from build123d import *

# Parameters (mm, degrees)
SKETCH1_W               = 107.35
SKETCH1_H               = 69.35
BOSS_EXTRUDE1_DEPTH     = 1.5875
CUT_EXTRUDE2_DEPTH      = 64.920899605
CUT_EXTRUDE2_DEPTH_BACK = 64.920899605
SKETCH2_R               = 1.5
SKETCH2_W               = 101
SKETCH2_H               = 42
SKETCH3_W               = 107.35
SKETCH3_H               = 69.35
SKETCH3_W_2             = 101
SKETCH3_H_2             = 63
BOSS_EXTRUDE2_DEPTH     = 40
SKETCH5_R               = 3.571875
CUT_EXTRUDE3_DEPTH      = 25.4
CUT_EXTRUDE4_DEPTH      = 121.232683914
SKETCH10_W              = 47.370876146
SKETCH10_H              = 31.5
CUT_EXTRUDE5_DEPTH      = 25.4
FILLET1_R               = 1.5


with BuildPart() as part:
    # Sketch1 → Boss-Extrude1 (new, symmetric)
    with BuildSketch(Plane.XY):
        Rectangle(SKETCH1_W, SKETCH1_H)
    extrude(amount=BOSS_EXTRUDE1_DEPTH, both=True)

    # Sketch2 → Cut-Extrude2 (cut, two sides: drawn at the far end of the back side and taken through both)
    with BuildSketch(Plane.XY.offset(-CUT_EXTRUDE2_DEPTH_BACK)):
        with Locations((-46.5, 27.5)):
            Circle(SKETCH2_R)
        with Locations((46.5, 27.5)):
            Circle(SKETCH2_R)
        with Locations((46.5, -27.5)):
            Circle(SKETCH2_R)
        with Locations((-46.5, -27.5)):
            Circle(SKETCH2_R)
        Rectangle(SKETCH2_W, SKETCH2_H)
    extrude(amount=CUT_EXTRUDE2_DEPTH + CUT_EXTRUDE2_DEPTH_BACK, mode=Mode.SUBTRACT)

    # Sketch3 → Boss-Extrude2 (add)
    with BuildSketch(Plane(origin=(0, 0, -1.5875), x_dir=(-1, 0, 0), z_dir=(0, 0, -1))):
        Rectangle(SKETCH3_W, SKETCH3_H)
        Rectangle(SKETCH3_W_2, SKETCH3_H_2, mode=Mode.SUBTRACT)
    extrude(amount=BOSS_EXTRUDE2_DEPTH)

    # Sketch5 → Cut-Extrude3 (cut)
    with BuildSketch(Plane(origin=(0, -31.5, 0), x_dir=(1, 0, 0), z_dir=(0, 1, 0))):
        with Locations(Location((0, 31.5875, 0), (0, 0, 270))):
            Circle(SKETCH5_R)
    extrude(amount=-CUT_EXTRUDE3_DEPTH, mode=Mode.SUBTRACT)

    # Sketch8 → Cut-Extrude4 (cut, through all)
    with BuildSketch(Plane.ZY.offset(53.675)):
        Polygon((-23.5875, 34.675), (-41.5875, -31.5), (-41.5875, 34.675), align=None)
    extrude(amount=-CUT_EXTRUDE4_DEPTH, mode=Mode.SUBTRACT)

    # Sketch10 → Cut-Extrude5 (cut)
    with BuildSketch(Plane(origin=(-50.5, 0, 0), x_dir=(0, 0, -1), z_dir=(1, 0, 0))):
        with Locations((25.272938073, 15.75)):
            Rectangle(SKETCH10_W, SKETCH10_H)
    extrude(amount=-CUT_EXTRUDE5_DEPTH, mode=Mode.SUBTRACT)

    # Fillet1
    fillet1_edges = [part.edges().sort_by_distance(p)[0] for p in [
        (-53.675, 0, 1.5875),
        (-53.675, -33.0875, -41.5875),
        (53.675, 0, 1.5875),
        (53.675, -33.0875, -41.5875),
        (-53.675, 34.675, -11),
        (53.675, 34.675, -11),
        (53.675, 1.5875, -32.5875),
        (0, 34.675, -23.5875),
        (-53.675, -15.75, -37.303404798),
        (0, 34.675, 1.5875),
        (-53.675, 33.0875, -24.019309596),
    ]]
    fillet(fillet1_edges, radius=FILLET1_R)


solid = part.part
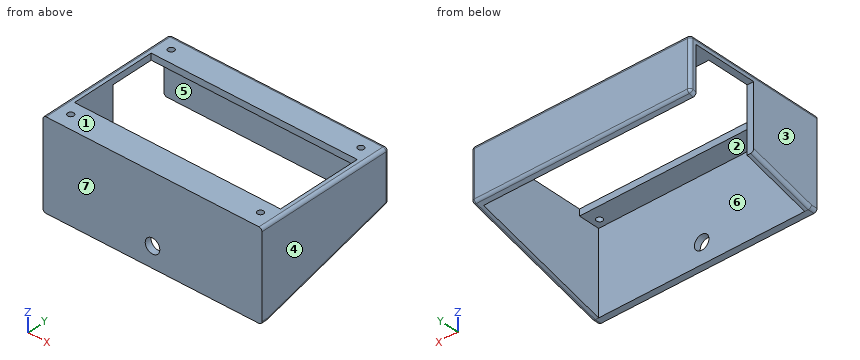
Source: CAD feature listing. Evaluate the final solid. Frame: model axes, mm. Face numbers are marked on the shaded views. A direction names the side the tool comes from. Round coordinates to 2 decimals unless told otherwise and drop trailing zeros. Loops run counter-clockwise (first coordinate to the right, second up) from the corner with the lowest first, then second, coordinate; pieces in that order, holes last. Notation, with made-up numbers: M 26.25,37.5 L 47.25,37.5 A29 cw 47.25,59.5 Z; hole C -31.75,-2 d9. An arc over 180 degrees is marked long. Return JSON: item names as keys, results as strings. Group by question number.
1. Material intervals for line 1 along Y through (x, z) = (-46.5, -0.1) (3 decimals); line 2 along Y through (x, z) = (4, -0.5) (3 decimals); line 3 along Y through (x, z) = (-15.5, -5) (3 decimals), sorted ascending. Write a range as from..to.
2. Section query B-B on x = -28.5. Output: boundary loops of the cut face in (y, z) (1 decimal).
3. Section query D-D on x = -46.5. Output: boundary loops of the cut face in (y, z) (1 decimal).
4. Reachability of the marked faces 5, 6 and 7 from +Z, -Z, +X, -X, +Y, -Y: full face, straight path, thin tool, end or side. Return the list, or none.
5. Section query C-C on z = -10. Output: boundary loops of the cut face in (x, y) (3 decimals), and give its area (3 significant figures).
6. Section query A-A on x = 0. Output: boundary loops of the cut face in (y, z) (1 decimal).
7. Pin query (flat end, axial travel): pin 1 (11.5 mm diameter, centred on x = 0, z = -31.59, fed in from +Y). Return the tip coordinate at first contact, or that it passes through.
8. Mould query, pull axis X, two halves, no side actions, for the marked faces 1, 2, 3 and 4. Classes: released by +X, released by -X, zero draft, split by the parting line, or undercut.
Checks:
{
 "1": {"line 1": "y = -34.675..-29, -26..-21, 21..26, 29..34.675", "line 2": "y = -34.675..-21, 21..34.675", "line 3": "y = -34.675..-31.5, 31.5..34.675"},
 "2": {"outline": "M -34.7,-41.6 L -31.5,-41.6 L -31.5,-1.6 L -21,-1.6 L -21,1.6 L -34.7,1.6 Z; M 21,-1.6 L 31.5,-1.6 L 31.5,-24.5 L 33.6,-23.9 A1.5 ccw 34.7,-22.4 L 34.7,0.1 A1.5 ccw 33.2,1.6 L 21,1.6 Z"},
 "3": {"outline": "M -34.7,-41.6 L -31.5,-41.6 L -31.5,-1.6 L -29,-1.6 L -29,1.6 L -34.7,1.6 Z; M -26,-1.6 L -21,-1.6 L -21,1.6 L -26,1.6 Z; M 21,-1.6 L 26,-1.6 L 26,1.6 L 21,1.6 Z; M 29,-1.6 L 31.5,-1.6 L 31.5,-24.5 L 33.6,-23.9 A1.5 ccw 34.7,-22.4 L 34.7,0.1 A1.5 ccw 33.2,1.6 L 29,1.6 Z"},
 "4": {"face 5": "-Z, -X", "face 6": "-Z", "face 7": "+Z, -Z, +X, -X, -Y"},
 "5": {"outline": "M -53.675,-34.675 L 53.675,-34.675 L 53.675,33.175 A1.5 ccw 52.175,34.675 L -52.175,34.675 A1.5 ccw -53.675,33.175 L -53.675,31.5 L 50.5,31.5 L 50.5,-31.5 L -50.5,-31.5 L -50.5,0 L -53.675,0 Z", "area": "981 mm²"},
 "6": {"outline": "M -34.7,-41.6 L -31.5,-41.6 L -31.5,-35.2 L -34.7,-35.2 Z; M -34.7,-28 L -31.5,-28 L -31.5,-1.6 L -21,-1.6 L -21,1.6 L -34.7,1.6 Z; M 21,-1.6 L 31.5,-1.6 L 31.5,-24.5 L 33.6,-23.9 A1.5 ccw 34.7,-22.4 L 34.7,0.1 A1.5 ccw 33.2,1.6 L 21,1.6 Z"},
 "7": {"pin 1": "stops at y = -31.5"},
 "8": {"face 1": "zero draft", "face 2": "undercut", "face 3": "released by -X", "face 4": "released by +X"}
}
